```python
from build123d import *

# Parameters (mm, degrees)
F1_DEPTH = 9.525
F2_W     = 9.525
F2_H     = 6.35
F3_DEPTH = 528.321


with BuildPart() as f1:
    # F0 (on Front) → F1 (new body, symmetric)
    with BuildSketch(Plane.XZ):
        Polygon((254, 149.225), (-254, 149.225), (-254, 118.745), (-274.32, 118.745), (-274.32, 80.645), (-254, 80.645), (-254, 19.05), (-274.32, 19.05), (-274.32, -19.05), (-254, -19.05), (-254, -80.645), (-274.32, -80.645), (-274.32, -118.745), (-254, -118.745), (-254, -149.225), (254, -149.225), (254, -118.745), (274.32, -118.745), (274.32, -80.645), (254, -80.645), (254, -19.05), (274.32, -19.05), (274.32, 19.05), (254, 19.05), (254, 80.645), (274.32, 80.645), (274.32, 118.745), (254, 118.745), align=None)
    extrude(amount=F1_DEPTH, both=True)

    # F2 (on face) → F3 (cut, through all)
    with BuildSketch(Plane(origin=(-254, 0, 0), x_dir=(0, -1, 0), z_dir=(-1, 0, 0))):
        with Locations((4.7625, -146.05)):
            Rectangle(F2_W, F2_H)
    extrude(amount=-F3_DEPTH, mode=Mode.SUBTRACT)


solid = f1.part
```
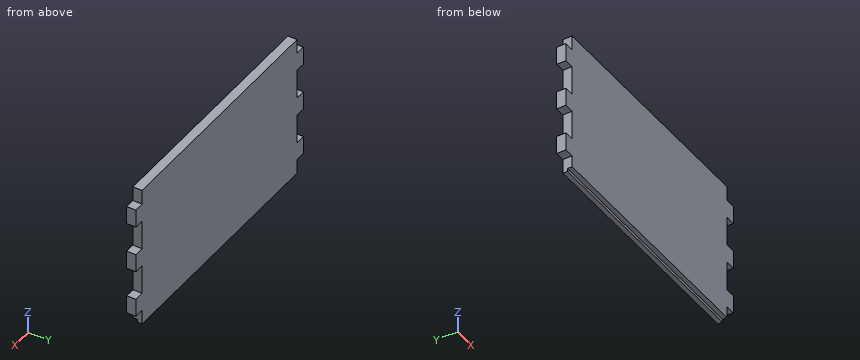
Input: part model. Units: mm. Frame: model coordinates. Give positions to 0.01 mm unless a question says otherwise; leave off trailing zeros. Order: outer loops, then holes, each group sorted by start corner. A loop starts at its lowest first (then second) coordinate and runs counter-clockwise, first axis right, second up.
1. Pin query (flat end, axial travel): pin 1 (9.5 mm diameter, centred on x = -263, y = -3.5, fed in from -Z) (3 decimals); pin 2 (5.5 mm diameter, centred on y = -3.5, z = 131.5, fed in from +X); pin 3 (4 mm diameter, centred on y = -0.5, z = 56, fed in from -X). Return the tip coordinate at first contact, or that it passes through.
Derived:
pin 1: stops at z = -118.745
pin 2: stops at x = 254
pin 3: stops at x = -254
2. Section B-B on z = 59. Return the cut outline in (x, y) (3 decimals), and give its area (3 significant figures).
Derived:
outline: (-254, -9.525) - (254, -9.525) - (254, 9.525) - (-254, 9.525) - close
area: 9,680 mm2
3. Section A-A on y = -3.25. Return the cut outline in (x, z) (3 decimals), and give its area (3 significant figures).
Derived:
outline: (-274.32, -118.745) - (-254, -118.745) - (-254, -142.875) - (254, -142.875) - (254, -118.745) - (274.32, -118.745) - (274.32, -80.645) - (254, -80.645) - (254, -19.05) - (274.32, -19.05) - (274.32, 19.05) - (254, 19.05) - (254, 80.645) - (274.32, 80.645) - (274.32, 118.745) - (254, 118.745) - (254, 149.225) - (-254, 149.225) - (-254, 118.745) - (-274.32, 118.745) - (-274.32, 80.645) - (-254, 80.645) - (-254, 19.05) - (-274.32, 19.05) - (-274.32, -19.05) - (-254, -19.05) - (-254, -80.645) - (-274.32, -80.645) - close
area: 153,000 mm2
4. Material intervals for L1, parallel to X at y = 4.75, z = -68; L2, parallel to Z at x = 216.5, y = -0.25 (3 decimals), sorted ascending.
Derived:
L1: x = -254 to 254
L2: z = -142.875 to 149.225
